from build123d import *

# Parameters (mm, degrees)
CROQUIS1_W              = 3
CROQUIS1_H              = 19.8
SALIENTE_EXTRUIR1_DEPTH = 7.5
CROQUIS2_W              = 3
CROQUIS2_H              = 1.42
SALIENTE_EXTRUIR2_DEPTH = 3
CROQUIS3_R              = 2.2
CORTAR_EXTRUIR1_DEPTH   = 3


with BuildPart() as part:
    # Croquis1 → Saliente-Extruir1 (new body)
    with BuildSketch(Plane.XY):
        Rectangle(CROQUIS1_W, CROQUIS1_H)
    extrude(amount=SALIENTE_EXTRUIR1_DEPTH)

    # Croquis2 → Saliente-Extruir2 (add)
    with BuildSketch(Plane(origin=(0, 0, 0), x_dir=(-1, 0, 0), z_dir=(0, 0, -1))):
        with Locations((0, 8.49)):
            Rectangle(CROQUIS2_W, CROQUIS2_H)
        with Locations((0, -8.49)):
            Rectangle(CROQUIS2_W, CROQUIS2_H)
    extrude(amount=SALIENTE_EXTRUIR2_DEPTH)

    # Croquis3 → Cortar-Extruir1 (cut)
    with BuildSketch(Plane.ZY.offset(1.5)):
        with Locations((2.91, -5.02)):
            Circle(CROQUIS3_R)
        with Locations((2.91, 5.02)):
            Circle(CROQUIS3_R)
    extrude(amount=-CORTAR_EXTRUIR1_DEPTH, mode=Mode.SUBTRACT)


solid = part.part
The model under review builds one solid part; all positions refer to its coordinate system, in mm. A direction names the side the tool comes from. Round coordinates to 2 decimals unless told otherwise and drop trailing zeros. Write each loop counter-clockwise with the first axis right and the second up, starting at its lowest first coordinate (ties: lowest second). Pieces come first, ordered by that corner, then holes. Notation, with made-up numbers: (-25.5, -37) -> (0.5, -37) arc R23 ccw to (0.5, -17) -> close; hole circle Ø6 at (79.25, -16). An arc over 180 degrees is marked (long way). Answer as a JSON object with one key per item and string values.
1. We need section D-D on y = -2. State the section outline as (x, z) points, and give its area (3 significant figures).
Results found:
{"outline": "(-1.5, 0) -> (1.5, 0) -> (1.5, 7.5) -> (-1.5, 7.5) -> close", "area": "22.5 mm^2"}
2. We need section C-C on z = 3.5. State the section outline as (x, y) points.
Results found:
{"outline": "(-1.5, -9.9) -> (1.5, -9.9) -> (1.5, -7.14) -> (-1.5, -7.14) -> close; (-1.5, -2.9) -> (1.5, -2.9) -> (1.5, 2.9) -> (-1.5, 2.9) -> close; (-1.5, 7.14) -> (1.5, 7.14) -> (1.5, 9.9) -> (-1.5, 9.9) -> close"}
3. We need section B-B on x = 0.9. State the section outline as (y, z) points.
Results found:
{"outline": "(-9.9, 0) -> (-9.2, 0) -> (-9.2, -3) -> (-7.78, -3) -> (-7.78, 0) -> (7.78, 0) -> (7.78, -3) -> (9.2, -3) -> (9.2, 0) -> (9.9, 0) -> (9.9, 7.5) -> (-9.9, 7.5) -> close; hole circle Ø4.4 at (-5.02, 2.91); hole circle Ø4.4 at (5.02, 2.91)"}
4. We need section A-A on y = -5.02. State the section outline as (x, z) points.
Results found:
{"outline": "(-1.5, 0) -> (1.5, 0) -> (1.5, 0.71) -> (-1.5, 0.71) -> close; (-1.5, 5.11) -> (1.5, 5.11) -> (1.5, 7.5) -> (-1.5, 7.5) -> close"}
5. Clearance check with flat-ended pins moving along their axes: pin 1 (1.5 mm diameter, centred on x = 0, z = -1, fed in from +Y); pin 2 (0.9 mm diameter, centred on x = 0, y = -2.5, fed in from -Z); pin 3 (0.9 mm diameter, centred on x = 0.5, z = -1, fed in from -Y). State where each tip first meets the part, or that it passes through.
Results found:
{"pin 1": "stops at y = 9.2", "pin 2": "stops at z = 0", "pin 3": "stops at y = -9.2"}
6. Machinability: for faces 1 (the face through (-0.021, -6.359, 1.164)), 2 (the face through (0, 9.2, -1)), 3 (the face through (0, -7.78, -1)), 4 (the face through (0, -8, -3)), 5 (the face through (0, -9.2, -1)), which of the approach directions +Z, -Z, +X, -X, +Y, -Y give a long, thin tool a straight path to every point of the face, cutting with its end or side? Answer none if there is none.
Results found:
{"face 1": "+X, -X", "face 2": "-Z, +X, -X, +Y", "face 3": "-Z, +X, -X", "face 4": "-Z, +X, -X, +Y, -Y", "face 5": "-Z, +X, -X, -Y"}
7. The part is to be moulded in two halves that separate along Z. For faces 6 (the face through (0, 0, 0)), 7 (the face through (0, 0, 7.5)), 8 (the face through (-0.021, 3.681, 1.164)), 9 (the face through (0, 9.9, 4)), say which applies: pulls with the +Z half, pulls with the -Z half, needs draft (parallel to the pull), parting line crosses it, or undercut.
Results found:
{"face 6": "pulls with the -Z half", "face 7": "pulls with the +Z half", "face 8": "undercut", "face 9": "needs draft"}
8. To check wall thickness, follow line 1 along Y through (x, z) = (0.2, 2.91); line 2 along Y through (x, z) = (0.6, -1.25); line 3 along Y through (x, z) = (-0.4, 2.25). State the ranges of each line that lie inside material, in increasing order.
Results found:
{"line 1": "y = -9.9 to -7.22, -2.82 to 2.82, 7.22 to 9.9", "line 2": "y = -9.2 to -7.78, 7.78 to 9.2", "line 3": "y = -9.9 to -7.12, -2.92 to 2.92, 7.12 to 9.9"}
